Can you work these out from the model? Positions are in its coordinate system, mm. A direction names the side the tool comes from. Round coordinates to 2 decimals unless told otherwise and drop trailing zeros. Order: outer loops, then holes, each group sorted by start corner. A loop starts at its lowest first (then second) coordinate and runs counter-clockwise, first axis right, second up.
Q1. For faces 4 (the face through (14.25, 17, 0)), 5 (the face through (-2.38, 35.79, -10.74)), 6 (the face through (-2, 44, 0)), which set-ups out of +Z, -Z, +X, -X, +Y, -Y let a thin tool reach every point of the face, with its end or its side?
Q2. If we section it at B-B (z = 0): Please give me the cut outline in (x, y), plus the area to 3 significant figures.
Q3. If we section it at C-C (y = 46.5): Please give me the cut outline in (x, z).
Q4. If I drill on line 1 (X direction, y = 34.1, z = 11.5); line 2 (Z direction, x = -11.5, y = 32.7) (3 decimals); line 3 (Y direction, x = 7, z = -9.5), over which ranges is the centre line in solid material (lowest first)?
Q5. We'd pull the mould along Z, two halves only. Please class faces 1 (the face through (-12, 31.5, -12)), 2 (the face through (-6, 35, 10)), 3 (the face through (0, 17, 14.075)): pulls with the +Z half, pulls with the -Z half, needs draft (parallel to the pull), parting line crosses it, or undercut.
Q6. If we section it at A-A (x = 0): Please give me the cut outline in (y, z) (3 decimals), plus the area to 3 significant figures.
Q7. Will these pins go through, and if not, where does the flat tip stop? P1, Ø1.2, axis at x = -12, z = -12, coming from the +Y side; P2, Ø0.8, axis at x = -11.5, z = 12, coming from the +Y side; P3, Ø1.5, axis at x = 4, z = -2, coming from the +Y side.
Q8. If we section it at D-D (z = 9.5): Please give me the cut outline in (x, y), plus the area to 3 significant figures.
Autodesk Inventor part; units mm, degrees
ref_plane "YZ Plane" through (0, 0, 0) normal (1, 0, 0) x (0, 1, 0)
ref_plane "XZ Plane" through (0, 0, 0) normal (0, 1, 0) x (-1, 0, 0)
ref_plane "XY Plane" through (0, 0, 0) normal (0, 0, 1) x (1, 0, 0)
sketch "草圖1" plane through (0, 0, 0) normal (0, 1, 0) x (-1, 0, 0)
  line L0 (-14.25, 14.075) -> (14.25, 14.075)
  line L1 (14.25, 14.075) -> (14.25, -14.075)
  line L2 (14.25, -14.075) -> (-14.25, -14.075)
  line L3 (-14.25, -14.075) -> (-14.25, 14.075)
  line L4 (-14.25, 14.075) -> (14.25, -14.075) construction
  line L5 (14.25, 14.075) -> (-14.25, -14.075) construction
  point P0 (0, 0)
  dimension "d0" = 28.5
  dimension "d1" = 28.15
extrude "擠出1" add sketch "草圖1" along normal blind 35
sketch "草圖2" plane through (0, 35, 0) normal (0, 1, 0) x (1, 0, 0)
  circle A0 centre (0, 0) radius 11
  dimension "d4" = 22
extrude "擠出2" add sketch "草圖2" along normal blind 1.6
sketch "草圖3" plane through (0, 36.6, 0) normal (0, 1, 0) x (1, 0, 0)
  arc A0 (-2, -1.5) -> (-2, 1.5) centre (0, 0) ccw
  line L0 (-2, -1.5) -> (-2, 1.5)
  dimension "d7" = 5
  dimension "d8" = 2
extrude "擠出3" add sketch "草圖3" along normal blind 15.4
sketch "草圖4" plane through (0, 35, 0) normal (0, 1, 0) x (1, 0, 0)
  line L0 (11.5, -11.5) -> (-11.5, -11.5) construction
  line L1 (-11.5, -11.5) -> (-11.5, 11.5) construction
  line L2 (-11.5, 11.5) -> (11.5, 11.5) construction
  line L3 (11.5, 11.5) -> (11.5, -11.5) construction
  arc A0 (-2, -1.5) -> (-2, 1.5) centre (0, 0) ccw construction
  line L4 (11.5, -11.5) -> (-11.5, 11.5) construction
  line L5 (-11.5, -11.5) -> (11.5, 11.5) construction
  circle A1 centre (-11.5, 11.5) radius 1.25
  circle A2 centre (-11.5, -11.5) radius 1.25
  circle A3 centre (11.5, -11.5) radius 1.25
  circle A4 centre (11.5, 11.5) radius 1.25
  dimension "d11" = 23
  dimension "d12" = 23
  dimension "d13" = 2.5
  dimension "d16" = 360
extrude "擠出4" cut sketch "草圖4" against normal blind 3.5
fillet "圓角1" radius 2 4 edges at (14.25, 17.5, 14.075) (14.25, 17.5, -14.075) (-14.25, 17.5, 14.075) (-14.25, 17.5, -14.075)
sketch "草圖5" plane through (0, 52, 0) normal (0, 1, 0) x (1, 0, 0)
  arc A0 (-2, -1.5) -> (-2, 1.5) centre (0, 0) ccw
properties part number "nema 11x35"
Solution:
1. face 4: +Z, -Z, +X, +Y, -Y
1. face 5: +Y
1. face 6: +Z, -Z, -X, +Y
2. outline: (-14.25, 0) - (14.25, 0) - (14.25, 35) - (11, 35) - (11, 36.6) - (2.5, 36.6) - (2.5, 52) - (-2, 52) - (-2, 36.6) - (-11, 36.6) - (-11, 35) - (-14.25, 35) - close
2. area: 1,100 mm2
3. outline: (-2, -1.5) arc R2.5 ccw (long way) to (-2, 1.5) - close
4. line 1: x = -14.25 to -12.75, -10.25 to 10.25, 12.75 to 14.25
4. line 2: z = -14.075 to -12.75, -10.25 to 10.25, 12.75 to 14.075
4. line 3: y = 0 to 35
5. face 1: undercut
5. face 2: needs draft
5. face 3: pulls with the +Z half
6. outline: (0, -14.075) - (35, -14.075) - (35, -11) - (36.6, -11) - (36.6, -2.5) - (52, -2.5) - (52, 2.5) - (36.6, 2.5) - (36.6, 11) - (35, 11) - (35, 14.075) - (0, 14.075) - close
6. area: 1,100 mm2
7. P1: stops at y = 35
7. P2: stops at y = 31.5
7. P3: stops at y = 36.6
8. outline: (-14.25, 0) - (14.25, 0) - (14.25, 35) - (5.55, 35) - (5.55, 36.6) - (-5.55, 36.6) - (-5.55, 35) - (-14.25, 35) - close
8. area: 1,020 mm2
